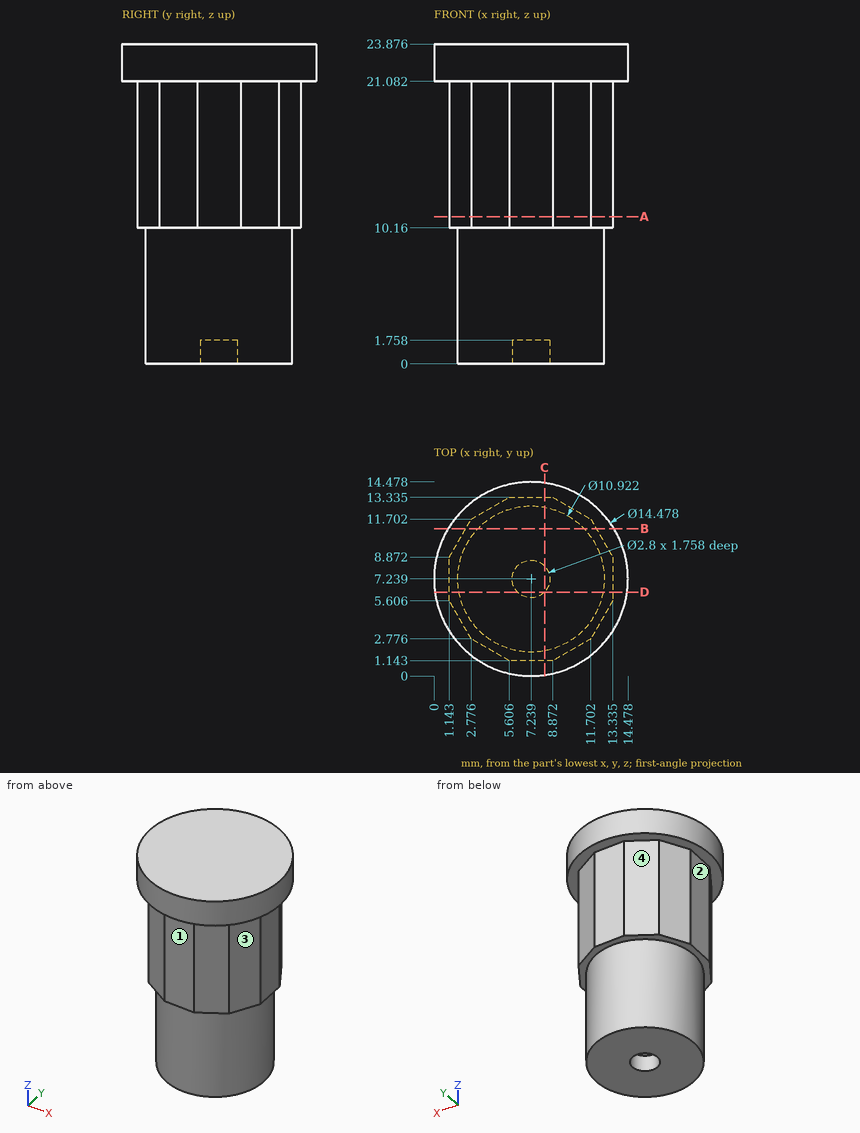
Print and shaded views of the part. All mm, measured from the part's lowest x, y and z. A direction names the side the tool comes from. Round coordinates to 2 decimals unless told otherwise and drop trailing zeros. Loops run counter-clockwise (first coordinate to the right, second up) from the corner with the lowest first, then second, coordinate; pieces in that order, holes last. Notation, with made-up numbers: (17, 11) -> (45, 11) arc R31 cw to (45, 48) -> close; hole circle Ø7 at (20.25, -3). An arc over 180 degrees is marked (long way). Use CSV: the item, a comma, the result in double quotes. Start each with the question number.
1) Cut at A-A, the plane z = 11. Write the cut outline in (x, y) (1 decimal).
2) Cut at B-B, the plane y = 11. Write the cut outline in (x, z) (1 decimal), plus the area to 3 significant figures.
3) Which spindle directions (+Z, -Z, +X, -X, +Y, -Y) get a long thin tool onto all of the face, cutting with end or side? Do the marked faces 1, 2, 3 and 4. Say none if no direction does.
4) Cut at D-D, the plane y = 6.25. Write the cut outline in (x, z) (1 decimal).
5) Cut at C-C, the plane x = 8.25. Write the cut outline in (y, z) (1 decimal), plus the area to 3 significant figures.
6) Drop flat-ended pins along their axis: P1, Ø2.5, axis at x = 7.239, y = 7.239, coming from the -Z side; P2, Ø3, axis at y = 8.5, z = 12.5, coming from the -X side; P3, Ø2.5, axis at x = 7.5, z = 14, coming from the +Y side (1 decimal). Give the stop position or say it passes through.
7) Wall check: L1, parallel to X at y = 7.25, z = 7.5; L2, parallel to X at y = 6.5, z = 14.75 (1 decimal); L3, parallel to Z at x = 5.5, y = 12.75 (1 decimal). Give the ranges that are in metal, low to high. Write a range as [from, to].
Determined:
1,outline,"(1.1, 5.6) -> (2.8, 2.8) -> (5.6, 1.1) -> (8.9, 1.1) -> (11.7, 2.8) -> (13.3, 5.6) -> (13.3, 8.9) -> (11.7, 11.7) -> (8.9, 13.3) -> (5.6, 13.3) -> (2.8, 11.7) -> (1.1, 8.9) -> close"
2,outline,"(1.1, 21.1) -> (2.4, 21.1) -> (2.4, 10.2) -> (3.3, 10.2) -> (3.3, 0) -> (11.2, 0) -> (11.2, 10.2) -> (12.1, 10.2) -> (12.1, 21.1) -> (13.4, 21.1) -> (13.4, 23.9) -> (1.1, 23.9) -> close"
2,area,"221 mm2"
3,face 1,"-Z, +X, -X, -Y"
3,face 2,"-Z, -X, +Y, -Y"
3,face 3,"-Z, +X, -Y"
3,face 4,"-Z, -X, +Y"
4,outline,"(0.1, 21.1) -> (1.1, 21.1) -> (1.1, 10.2) -> (1.9, 10.2) -> (1.9, 0) -> (6.2, 0) -> (6.2, 1.8) -> (8.2, 1.8) -> (8.2, 0) -> (12.6, 0) -> (12.6, 10.2) -> (13.3, 10.2) -> (13.3, 21.1) -> (14.4, 21.1) -> (14.4, 23.9) -> (0.1, 23.9) -> close"
5,outline,"(0.1, 21.1) -> (1.1, 21.1) -> (1.1, 10.2) -> (1.9, 10.2) -> (1.9, 0) -> (6.3, 0) -> (6.3, 1.8) -> (8.2, 1.8) -> (8.2, 0) -> (12.6, 0) -> (12.6, 10.2) -> (13.3, 10.2) -> (13.3, 21.1) -> (14.4, 21.1) -> (14.4, 23.9) -> (0.1, 23.9) -> close"
5,area,"279 mm2"
6,P1,"stops at z = 1.76"
6,P2,"stops at x = 1.14"
6,P3,"stops at y = 13.3"
7,L1,"x = [1.78, 12.7]"
7,L2,"x = [1.1, 13.3]"
7,L3,"z = [10.2, 23.9]"
